```python
from build123d import *

# Parameters (mm, degrees)
SKETCH1_R           = 1.6
SKETCH1_W           = 82.6
SKETCH1_H           = 61.2
BOSS_EXTRUDE1_DEPTH = 2
SKETCH2_W           = 84.6
SKETCH2_H           = 63.2
CUT_EXTRUDE1_DEPTH  = 1
CHAMFER1_SIZE       = 0.5
SKETCH3_R           = 2.9
CUT_EXTRUDE2_DEPTH  = 1
CHAMFER2_SIZE       = 0.5
CHAMFER3_SIZE       = 1
CUT_EXTRUDE3_DEPTH  = 0.8


with BuildPart() as part:
    # Sketch1 → Boss-Extrude1 (new body)
    with BuildSketch(Plane(origin=(0, 0, 0), x_dir=(1, 0, 0), z_dir=(0, 1, 0))):
        with BuildLine():
            Line((3, 0), (112, 0))
            ThreePointArc((112, 0), (114.121320344, 0.878679656), (115, 3))
            Line((115, 3), (115, 67))
            ThreePointArc((115, 67), (114.121320344, 69.121320344), (112, 70))
            Line((112, 70), (3, 70))
            ThreePointArc((3, 70), (0.878679656, 69.121320344), (0, 67))
            Line((0, 67), (0, 3))
            ThreePointArc((0, 3), (0.878679656, 0.878679656), (3, 0))
        make_face()
        with Locations((6.5, 63.5)):
            Circle(SKETCH1_R, mode=Mode.SUBTRACT)
        with Locations((6.5, 6.5)):
            Circle(SKETCH1_R, mode=Mode.SUBTRACT)
        with Locations((108.5, 6.5)):
            Circle(SKETCH1_R, mode=Mode.SUBTRACT)
        with Locations((108.5, 63.5)):
            Circle(SKETCH1_R, mode=Mode.SUBTRACT)
        with Locations((57.5, 35)):
            Rectangle(SKETCH1_W, SKETCH1_H, mode=Mode.SUBTRACT)
    extrude(amount=BOSS_EXTRUDE1_DEPTH)

    # Sketch2 → Cut-Extrude1 (cut)
    with BuildSketch(Plane.XZ):
        with Locations((57.5, -35)):
            Rectangle(SKETCH2_W, SKETCH2_H)
    extrude(amount=-CUT_EXTRUDE1_DEPTH, mode=Mode.SUBTRACT)

    # Chamfer1
    chamfer1_edges = [part.edges().sort_by_distance(p)[0] for p in [
        (16.2, 2, -35),
        (57.5, 2, -4.4),
        (98.8, 2, -35),
        (57.5, 2, -65.6),
    ]]
    chamfer(chamfer1_edges, length=CHAMFER1_SIZE)

    # Sketch3 → Cut-Extrude2 (cut)
    with BuildSketch(Plane(origin=(0, 2, 0), x_dir=(1, 0, 0), z_dir=(0, 1, 0))):
        with Locations((6.5, 63.5)):
            Circle(SKETCH3_R)
        with Locations((108.5, 63.5)):
            Circle(SKETCH3_R)
        with Locations((108.5, 6.5)):
            Circle(SKETCH3_R)
        with Locations((6.5, 6.5)):
            Circle(SKETCH3_R)
    extrude(amount=-CUT_EXTRUDE2_DEPTH, mode=Mode.SUBTRACT)

    # Chamfer2
    chamfer2_edges = [part.edges().sort_by_distance(p)[0] for p in [
        (105.6, 2, -63.5),
        (3.6, 2, -63.5),
        (3.6, 2, -6.5),
        (105.6, 2, -6.5),
    ]]
    chamfer(chamfer2_edges, length=CHAMFER2_SIZE)

    # Chamfer3
    chamfer3_edges = [part.edges().sort_by_distance(p)[0] for p in [
        (114.121320344, 2, -0.878679656),
        (115, 2, -35),
        (114.121320344, 2, -69.121320344),
        (57.5, 2, -70),
        (0.878679656, 2, -69.121320344),
        (0, 2, -35),
        (0.878679656, 2, -0.878679656),
        (57.5, 2, 0),
    ]]
    chamfer(chamfer3_edges, length=CHAMFER3_SIZE)

    # Sketch4 → Cut-Extrude3 (cut)
    with BuildSketch(Plane(origin=(0, 2, 0), x_dir=(1, 0, 0), z_dir=(0, 1, 0))):
        with BuildLine():
            Line((9.825395701, 30.960299483), (8.89586377, 33.118648479))
            ThreePointArc((8.89586377, 33.118648479), (8.290679151, 36.053871442), (7.685494532, 33.118648479))
            Line((7.685494532, 33.118648479), (6.755962601, 30.960299483))
            ThreePointArc((6.755962601, 30.960299483), (6.457149652, 31.104431492), (6.171741697, 31.273563139))
            Line((6.171741697, 31.273563139), (4.91328092, 30.43936643))
            Line((4.91328092, 30.43936643), (4.55972753, 30.792919821))
            Line((4.55972753, 30.792919821), (4.206174139, 31.146473212))
            Line((4.206174139, 31.146473212), (5.040370847, 32.404933989))
            ThreePointArc((5.040370847, 32.404933989), (4.706026565, 33.039059725), (4.494049066, 33.723871442))
            Line((4.494049066, 33.723871442), (3.014316768, 34.023871442))
            Line((3.014316768, 34.023871442), (3.014316768, 34.523871442))
            Line((3.014316768, 34.523871442), (3.014316768, 35.023871442))
            Line((3.014316768, 35.023871442), (4.494049066, 35.323871442))
            ThreePointArc((4.494049066, 35.323871442), (4.706026565, 36.00868316), (5.040370847, 36.642808896))
            Line((5.040370847, 36.642808896), (4.206174139, 37.901269673))
            Line((4.206174139, 37.901269673), (4.55972753, 38.254823064))
            Line((4.55972753, 38.254823064), (4.91328092, 38.608376454))
            Line((4.91328092, 38.608376454), (6.171741697, 37.774179746))
            ThreePointArc((6.171741697, 37.774179746), (6.805867433, 38.108524028), (7.490679151, 38.320501527))
            Line((7.490679151, 38.320501527), (7.790679151, 39.800233826))
            Line((7.790679151, 39.800233826), (8.290679151, 39.800233826))
            Line((8.290679151, 39.800233826), (8.790679151, 39.800233826))
            Line((8.790679151, 39.800233826), (9.090679151, 38.320501527))
            ThreePointArc((9.090679151, 38.320501527), (9.775490868, 38.108524028), (10.409616604, 37.774179746))
            Line((10.409616604, 37.774179746), (11.668077381, 38.608376454))
            Line((11.668077381, 38.608376454), (12.021630772, 38.254823064))
            Line((12.021630772, 38.254823064), (12.375184163, 37.901269673))
            Line((12.375184163, 37.901269673), (11.540987454, 36.642808896))
            ThreePointArc((11.540987454, 36.642808896), (11.875331737, 36.00868316), (12.087309236, 35.323871442))
            Line((12.087309236, 35.323871442), (13.567041534, 35.023871442))
            Line((13.567041534, 35.023871442), (13.567041534, 34.523871442))
            Line((13.567041534, 34.523871442), (13.567041534, 34.023871442))
            Line((13.567041534, 34.023871442), (12.087309236, 33.723871442))
            ThreePointArc((12.087309236, 33.723871442), (11.875331737, 33.039059725), (11.540987454, 32.404933989))
            Line((11.540987454, 32.404933989), (12.375184163, 31.146473212))
            Line((12.375184163, 31.146473212), (12.021630772, 30.792919821))
            Line((12.021630772, 30.792919821), (11.668077381, 30.43936643))
            Line((11.668077381, 30.43936643), (10.409616604, 31.273563139))
            ThreePointArc((10.409616604, 31.273563139), (10.12420865, 31.104431492), (9.825395701, 30.960299483))
        make_face()
    extrude(amount=-CUT_EXTRUDE3_DEPTH, mode=Mode.SUBTRACT)


solid = part.part
```
Source: CAD feature listing. Evaluate the final solid. Frame: model axes, mm. A direction names the side the tool comes from. Give positions to 0.01 mm unless a question says otherwise; leave off trailing zeros. Loops run counter-clockwise (first coordinate to the right, second up) from the corner with the lowest first, then second, coordinate; pieces in that order, holes last. Notation, with made-up numbers: (16.25, -37) - (39.25, -37) arc R21 cw to (39.25, -32) - close; hole circle Ø1 at (41, 61). An arc over 180 degrees is marked (long way). Use CSV: the item, a comma, the result in double quotes. Start each with the question number.
1. Section D-D (z = -6.5). Count the separate pieces of the cut face and the enclosed holes in it, then the cut area to 4 significant figures.
2. Draft query along Z for faces 3 (the conical face through (1.32, 1.6, -68.71)), 4 (the cylindrical face through (108.292, 0.493, -65.086)), 5 (the cylindrical face through (114.1, 0.49, -0.86)), 6 (the flat face through (57, 2, -2)). Return one class per face: +Z half, -Z half, draft (parallel to the pull), parting line (faces both ways), or undercut.
3. Pin query (flat end, axial travel): pin 1 (6.5 mm diameter, centred on x = 7, z = -7, fed in from +Y); pin 2 (3 mm diameter, centred on x = 6.5, z = -64, fed in from +Y). Return the tip coordinate at first contact, or that it passes through.
4. Section B-B (x = 108.5). Output: boundary loops of the cut face in (y, z).
5. Ray query, L1, parallel to Z at x = 108.5, y = 0.75; L2, parallel to X at y = 0.4, z = -63.5; L3, parallel to X at y = 0.85, z = -9. Return the intervals inside material, ascending.
6. Reachability of faces 1 (the flat face through (110, 1, -62)), 2 (the cylindrical face through (7.24, 0.49, -5.08)) from +Z, -Z, +X, -X, +Y, -Y: full face, straight path, thin tool, end or side. Return the list, or none.
7. Section C-C (z = -44). Output: boundary loops of the cut face in (x, y).
8. Section A-A (x = 27). Output: boundary loops of the cut face in (y, z).
Response:
1,separate pieces,"4"
1,enclosed holes,"0"
1,area,"43.05 mm²"
2,face 3,"-Z half"
2,face 4,"undercut"
2,face 5,"+Z half"
2,face 6,"draft"
3,pin 1,"y = 2"
3,pin 2,"y = 1"
4,outline,"(0, -70) - (1, -70) - (2, -69) - (2, -66.9) - (1.5, -66.4) - (1, -66.4) - (1, -65.1) - (0, -65.1) - close; (0, -61.9) - (1, -61.9) - (1, -60.6) - (1.5, -60.6) - (2, -60.1) - (2, -9.9) - (1.5, -9.4) - (1, -9.4) - (1, -8.1) - (0, -8.1) - close; (0, -4.9) - (1, -4.9) - (1, -3.6) - (1.5, -3.6) - (2, -3.1) - (2, -1) - (1, 0) - (0, 0) - close"
5,L1,"-70 to -65.1, -61.9 to -8.1, -4.9 to 0"
5,L2,"0 to 4.9, 8.1 to 15.2, 99.8 to 106.9, 110.1 to 115"
5,L3,"0 to 15.2, 99.8 to 115"
6,face 1,"+Y"
6,face 2,"+Y, -Y"
7,outline,"(0, 0) - (15.2, 0) - (15.2, 1) - (16.2, 1) - (16.2, 1.5) - (15.7, 2) - (1, 2) - (0, 1) - close; (98.8, 1) - (99.8, 1) - (99.8, 0) - (115, 0) - (115, 1) - (114, 2) - (99.3, 2) - (98.8, 1.5) - close"
8,outline,"(0, -70) - (1, -70) - (2, -69) - (2, -66.1) - (1.5, -65.6) - (1, -65.6) - (1, -66.6) - (0, -66.6) - close; (0, -3.4) - (1, -3.4) - (1, -4.4) - (1.5, -4.4) - (2, -3.9) - (2, -1) - (1, 0) - (0, 0) - close"
